The model under review builds one solid part; all positions refer to its coordinate system, in mm. Give positions to 0.01 mm unless a question says otherwise; leave off trailing zeros. Loops run counter-clockwise (first coordinate to the right, second up) from the corner with the lowest first, then second, coordinate; pieces in that order, holes last. Notation, with made-up numbers: (-32.5, -13) - (1.5, -13) arc R24 ccw to (1.5, 11) - close; hole circle Ø6 at (-37, 56). An arc over 180 degrees is marked (long way). Return JSON: item names as keys, results as strings. Group by question number.
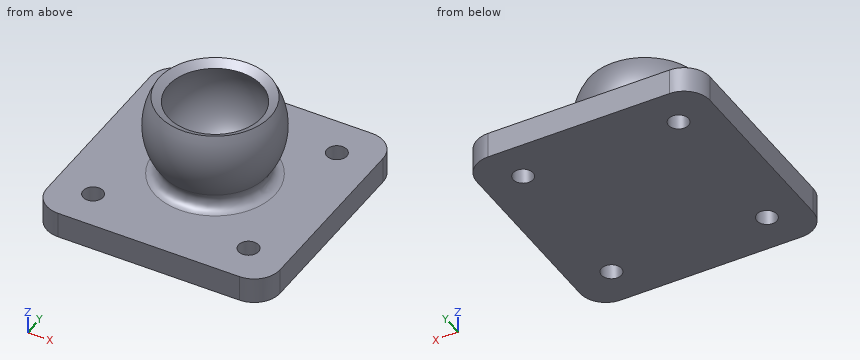
```python
from build123d import *

# Parameters (mm, degrees)
SKETCH1_W           = 45
SKETCH1_H           = 45
BOSS_EXTRUDE1_DEPTH = 5
FILLET1_R           = 5
SKETCH2_R           = 1.925
CUT_EXTRUDE1_DEPTH  = 33.210246817
FILLET2_R           = 2


with BuildPart() as part:
    # Sketch1 → Boss-Extrude1 (new body)
    with BuildSketch(Plane.XY):
        Rectangle(SKETCH1_W, SKETCH1_H)
    extrude(amount=BOSS_EXTRUDE1_DEPTH)

    # Fillet1
    fillet1_edges = [part.edges().sort_by_distance(p)[0] for p in [
        (22.5, -22.5, 2.5),
        (-22.5, -22.5, 2.5),
        (-22.5, 22.5, 2.5),
        (22.5, 22.5, 2.5),
    ]]
    fillet(fillet1_edges, radius=FILLET1_R)

    # Sketch2 → Cut-Extrude1 (cut, through all)
    with BuildSketch(Plane.XY.offset(5)):
        with Locations((15, 15)):
            Circle(SKETCH2_R)
        with Locations(Location((15, -15, 0), (0, 0, 180))):
            Circle(SKETCH2_R)
        with Locations((-15, -15)):
            Circle(SKETCH2_R)
        with Locations(Location((-15, 15, 0), (0, 0, 180))):
            Circle(SKETCH2_R)
    extrude(amount=-CUT_EXTRUDE1_DEPTH, mode=Mode.SUBTRACT)

    # Sketch3 → Revolve5 (revolve)
    with BuildSketch(Plane(origin=(0, 0, 0), x_dir=(1, 0, 0), z_dir=(0, 1, 0))):
        with BuildLine():
            Line((0, -3), (0, -5))
            ThreePointArc((0, -5), (10.3, -15.3), (0, -25.6))
            Line((0, -25.6), (0, -27.6))
            ThreePointArc((0, -27.6), (12.3, -15.3), (0, -3))
        make_face()
    revolve(axis=Axis((0, 0, 3), (0, 0, 1)))

    # Fillet2
    fillet2_edges = [part.edges().sort_by_distance(p)[0] for p in [
        (-6.723094526, 0, 5),
    ]]
    fillet(fillet2_edges, radius=FILLET2_R)

    # Cut-Revolve9: read off the stored shape, not the designer's step
    # Cut-Revolve9 outline → Cut-Revolve9 (revolve, cut)
    with BuildSketch(Plane.XZ):
        Polygon((9.008582984, 21.263158329), (9.008582984, 20.293539089), (10.757822398, 21.263158329), align=None)
    revolve(axis=Axis((0, 0, 0), (0, 0, 1)), mode=Mode.SUBTRACT)

    # Cut-Revolve9 2 outline → Cut-Revolve9 2 (revolve, cut)
    with BuildSketch(Plane.XZ):
        with BuildLine():
            Line((9.008582984, 21.263158329), (10.757822401, 21.263158323))
            ThreePointArc((10.757822401, 21.263158323), (6.242721867, 25.898038672), (0, 27.6))
            Line((0, 27.6), (0, 25.6))
            ThreePointArc((0, 25.6), (5.227645138, 24.174780353), (9.008582983, 20.293539089))
            Line((9.008582983, 20.293539089), (9.008582984, 21.263158329))
        make_face()
    revolve(axis=Axis((0, 0, 0), (0, 0, 1)), mode=Mode.SUBTRACT)


solid = part.part
```
1) We need section A-A, the plane y = 15. Write out the cut boundary in (x, z) (3 decimals), plus the area to 4 significant figures.
2) We need section C-C, the plane z = 3.75. Write out the cut boundary in (x, y) (3 decimals).
3) We need section D-D, the plane z = 19.5. Write out the cut boundary in (x, y).
4) To check wall thickness, follow line 1 (Y direction, x = 15, z = 3.65) (3 decimals); line 2 (Z direction, x = 3, y = -13.5); line 3 (Y direction, x = 0.5, z = 11.25). State the ranges of each line that lie inside material, in increasing order.
5) For pin 1 Ø3.5 at (x, y) = (-15, 15) entering from -Z; pin 2 Ø1 at (x, y) = (10.5, 0.5) entering from +Z; pin 3 Ø5 at (x, z) = (-6, 19) entering from -Y; pin 4 Ø6 at (x, y) = (-15, -15) entering from +Z, all flat-tipped, find the tip position at first contact; note any pin that passes through.
Findings:
{
 "1": {"outline": "(-22.5, 0) - (-16.925, 0) - (-16.925, 5) - (-22.5, 5) - close; (-13.075, 0) - (13.075, 0) - (13.075, 5) - (-13.075, 5) - close; (16.925, 0) - (22.5, 0) - (22.5, 5) - (16.925, 5) - close", "area": "186.5 mm^2"},
 "2": {"outline": "(-22.5, -17.5) arc R5 ccw to (-17.5, -22.5) - (17.5, -22.5) arc R5 ccw to (22.5, -17.5) - (22.5, 17.5) arc R5 ccw to (17.5, 22.5) - (-17.5, 22.5) arc R5 ccw to (-22.5, 17.5) - close; hole circle Ø3.85 at (-15, -15); hole circle Ø3.85 at (-15, 15); hole circle Ø3.85 at (15, -15); hole circle Ø3.85 at (15, 15)"},
 "3": {"outline": "circle Ø23.12 at (0, 0); hole circle Ø18.81 at (0, 0)"},
 "4": {"line 1": "y = -22.5 to -16.925, -13.075 to 13.075, 16.925 to 22.5", "line 2": "z = 0 to 5", "line 3": "y = -11.6 to -9.46, 9.46 to 11.6"},
 "5": {"pin 1": "passes through", "pin 2": "stops at z = 21.26", "pin 3": "stops at y = -11.43", "pin 4": "stops at z = 5"}
}
